Geometry: final body of the model. Coordinates: model frame, mm. Face numbers are marked on the shaded views. Round coordinates to 2 decimals unless told otherwise and drop trailing zeros. Loops run counter-clockwise (first coordinate to the right, second up) from the corner with the lowest first, then second, coordinate; pieces in that order, holes last. Notation, with made-up numbers: M 3.5,59.5 L 32.5,59.5 A28 ccw 32.5,79.5 Z; hole C 66,66.5 d6. An arc over 180 degrees is marked long. Return JSON: item names as keys, results as strings.
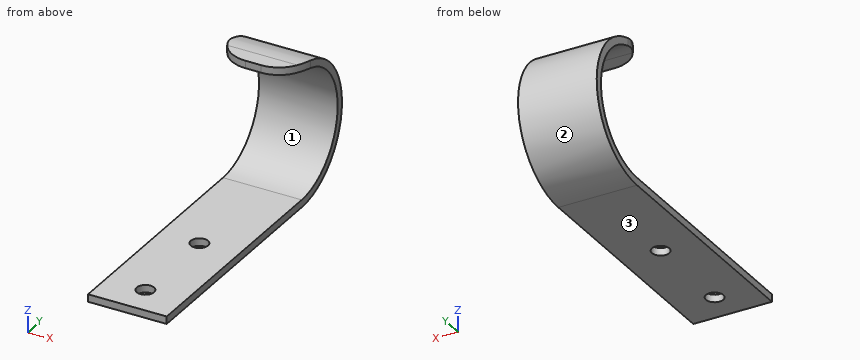
from build123d import *

# Parameters (mm, degrees)
BOSS_EXTRUDE1_DEPTH = 25
FILLET1_R           = 10
SKETCH2_R           = 2.75
CUT_EXTRUDE1_DEPTH  = 25


with BuildPart() as part:
    # Sketch1 → Boss-Extrude1 (new body)
    with BuildSketch(Plane(origin=(0, 0, 0), x_dir=(0, 0, -1), z_dir=(1, 0, 0))):
        with BuildLine():
            Line((0, 0), (0, 75))
            ThreePointArc((0, 75), (-20, 95), (-40, 75))
            Line((-40, 75), (-40, 70))
            Line((-40, 70), (-42.38, 70))
            Line((-42.38, 70), (-42.38, 75))
            ThreePointArc((-42.38, 75), (-20, 97.38), (2.38, 75))
            Line((2.38, 75), (2.38, 0))
            Line((2.38, 0), (0, 0))
        make_face()
    extrude(amount=BOSS_EXTRUDE1_DEPTH)

    # Fillet1
    fillet1_edges = [part.edges().sort_by_distance(p)[0] for p in [
        (0, 70, 41.19),
        (25, 70, 41.19),
    ]]
    fillet(fillet1_edges, radius=FILLET1_R)

    # Sketch2 → Cut-Extrude1 (cut)
    with BuildSketch(Plane.XY):
        with Locations((12.5, 10)):
            Circle(SKETCH2_R)
        with Locations((12.5, 40)):
            Circle(SKETCH2_R)
    extrude(amount=-CUT_EXTRUDE1_DEPTH, mode=Mode.SUBTRACT)


solid = part.part
Q1. Section query C-C (x = 6.5). Output: boundary loops of the cut face in (y, z), plus the area to 3 significant figures.
Determined:
{"outline": "M 0,-2.38 L 75,-2.38 A22.38 ccw 75,42.38 L 70.63,42.38 L 70.63,40 L 75,40 A20 cw 75,0 L 0,0 Z", "area": "347 mm^2"}
Q2. Material intervals for L1, parallel to Z at x = 9, y = 25; L2, parallel to Z at x = 12.5, y = 74; L3, parallel to Y at x = 12.5, z = -0.7, sorted ascending.
Determined:
{"L1": "z = -2.38 to 0", "L2": "z = -2.38 to 0, 40 to 42.38", "L3": "y = 0 to 7.25, 12.75 to 37.25, 42.75 to 83.51"}
Q3. Pull-direction query (Z, two-part tool) for the marked faces 1, 2 and 3; classes: pulls with the +Z half, pulls with the -Z half, needs draft (parallel to the pull), parting line crosses it, or undercut.
Determined:
{"face 1": "undercut", "face 2": "parting line crosses it", "face 3": "pulls with the -Z half"}
Q4. Pin query (flat end, axial travel): pin 1 (3 mm diameter, centred on x = 3.5, y = 43, fed in from +Z); pin 2 (6 mm diameter, centred on x = 10, z = 9.5, fed in from -Y); pin 3 (12 mm diameter, centred on x = 4, y = 68, fed in from +Z); pin 4 (5 mm diameter, centred on x = 12, z = 5, fed in from -Y). Return the tip coordinate at first contact, or that it passes through.
Determined:
{"pin 1": "stops at z = 0", "pin 2": "stops at y = 89.76", "pin 3": "stops at z = 42.38", "pin 4": "stops at y = 84.68"}
Q5. Section query A-A (x = 12.5). Output: boundary loops of the cut face in (y, z).
Determined:
{"outline": "M 0,-2.38 L 7.25,-2.38 L 7.25,0 L 0,0 Z; M 12.75,-2.38 L 37.25,-2.38 L 37.25,0 L 12.75,0 Z; M 42.75,-2.38 L 75,-2.38 A22.38 ccw 75,42.38 L 70,42.38 L 70,40 L 75,40 A20 cw 75,0 L 42.75,0 Z"}
Q6. Section query D-D (z = 20). Output: boundary loops of the cut face in (x, y), plus the area to 3 significant figures.
Determined:
{"outline": "M 0,95 L 25,95 L 25,97.38 L 0,97.38 Z", "area": "59.5 mm^2"}
Q7. Section query B-B (y = 10). Output: boundary loops of the cut face in (x, z), plus the area to 3 significant figures.
Determined:
{"outline": "M 0,-2.38 L 9.75,-2.38 L 9.75,0 L 0,0 Z; M 15.25,-2.38 L 25,-2.38 L 25,0 L 15.25,0 Z", "area": "46.4 mm^2"}
